Could you check a few things on this drawing? It's one solid part, dimensions in mm from its lowest x, y, z. Give positions to 0.01 mm unless a question says otherwise; leave off trailing zeros. Loops run counter-clockwise (first coordinate to the right, second up) from the corner with the lowest first, then second, coordinate; pieces in that order, holes last.
Q1. Thinking about a two-plate mould opening in X: for the marked faces 1 and 2, which applies, pulls with the +X half, pulls with the -X half, needs draft (parallel to the pull), parting line crosses it, or undercut?
Q2. I need wall thicknesses on probe 1 along Y at (x, z) = (3.5, 13); probe 2 along X at (y, z) = (1.75, 4.5); probe 3 along X at (y, z) = (4, 25.25). Which ranges of each line are inside material? Lowest first, please.
Q3. Suppose I cut it at A-A (y = 3.5). List the corners of the cut face in (x, z) for me, and give its area (3 significant figures).
Q4. Suppose I cut it at C-C (z = 11). List the corners of the cut face in (x, y) for me.
Q5. I'm going to push flat-ended pins straight in: P1, Ø1, axis at y = 4.5, z = 3, coming from the +X side; P2, Ø1.5, axis at x = 2.5, y = 2, coming from the -Z side; P3, Ø3, axis at y = 1, z = 10, coming from the -X side. Where does each tip first touch, or does it pass through?
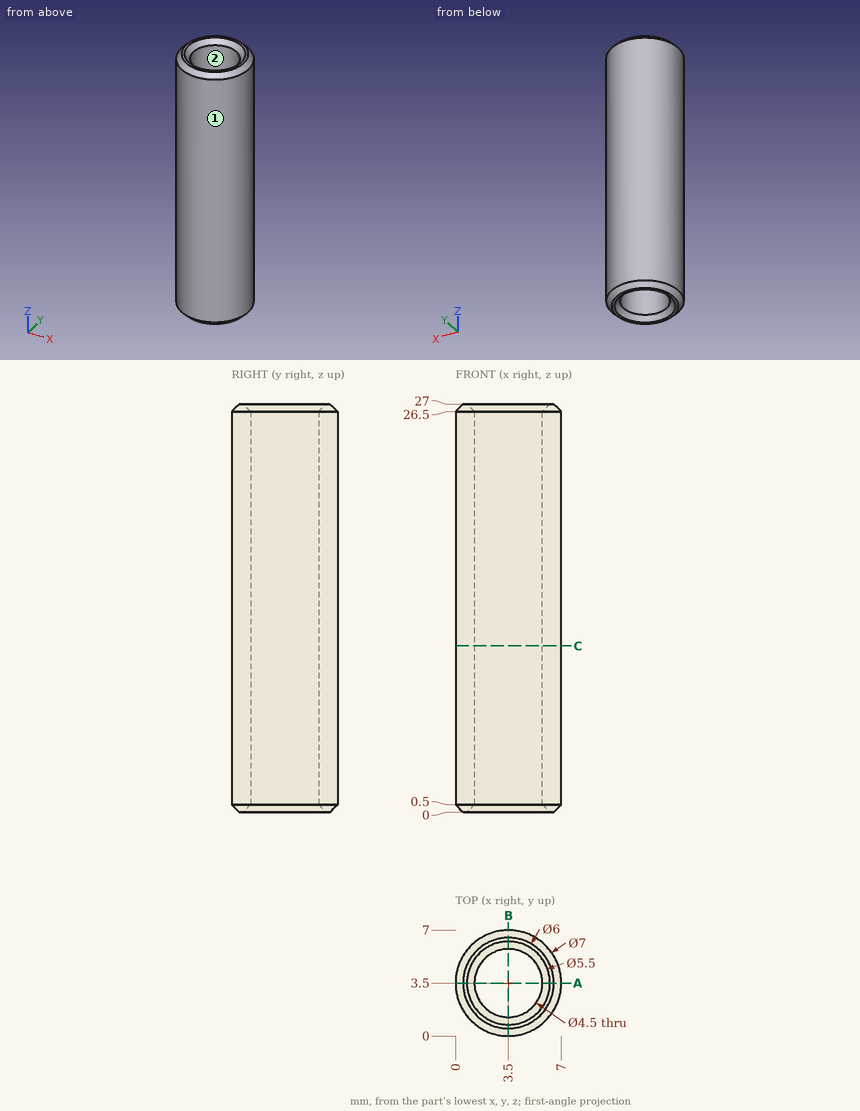
Solutions:
1. face 1: parting line crosses it
1. face 2: undercut
2. probe 1: y = 0 to 1.25, 5.75 to 7
2. probe 2: x = 0.47 to 2.09, 4.91 to 6.53
2. probe 3: x = 0.04 to 1.31, 5.69 to 6.96
3. outline: (0, 0.5) - (0.5, 0) - (0.75, 0) - (1.25, 0.5) - (1.25, 26.5) - (0.75, 27) - (0.5, 27) - (0, 26.5) - close; (5.75, 0.5) - (6.25, 0) - (6.5, 0) - (7, 0.5) - (7, 26.5) - (6.5, 27) - (6.25, 27) - (5.75, 26.5) - close
3. area: 66.5 mm2
4. outline: circle Ø7 at (3.5, 3.5); hole circle Ø4.5 at (3.5, 3.5)
5. P1: stops at x = 6.96
5. P2: stops at z = 0.2
5. P3: stops at x = 0.15
